```python
from build123d import *

# Parameters (mm, degrees)
SKETCH037_R     = 2.45
PAD019_DEPTH    = 1.6
SKETCH038_R     = 2.45
PAD020_DEPTH    = 1.6
SKETCH062_W     = 1.7771358599
SKETCH062_H     = 3.8
POCKET024_DEPTH = 1.6


with BuildPart() as part:
    # Sketch037 → Pad019 (new body)
    with BuildSketch(Plane.YZ.offset(-8.7)):
        with BuildLine():
            ThreePointArc((-6, 6), (-7.4371881489, -9.1), (-6, -24.2))
            Line((-6, -24.2), (0, -24.2))
            ThreePointArc((0, -24.2), (4.2426406871, -22.4426406871), (6, -18.2))
            Line((6, 0), (6, -18.2))
            ThreePointArc((6, 0), (4.2426406871, 4.2426406871), (0, 6))
            Line((-6, 6), (0, 6))
        make_face()
        Circle(SKETCH037_R, mode=Mode.SUBTRACT)
        with Locations((0, -18.2)):
            Circle(SKETCH037_R, mode=Mode.SUBTRACT)
    extrude(amount=PAD019_DEPTH)

    # Sketch038 → Pad020 (join)
    with BuildSketch(Plane.YZ.offset(-8.7)):
        with BuildLine():
            ThreePointArc((5.8114989668, -16.707860677), (3.6774423219, -13.4590699257), (0, -12.2))
            Line((-7.3771358599, -12.2), (0, -12.2))
            ThreePointArc((-6, 6), (-7.2090239265, -3.0606187573), (-7.3771358599, -12.2))
            Line((-6, 6), (0, 6))
            ThreePointArc((6, 0), (4.2426406871, 4.2426406871), (0, 6))
            Line((6, 0), (6, -17.4420237293))
            Line((6, -17.4420237293), (5.8114989668, -16.707860677))
        make_face()
        Circle(SKETCH038_R, mode=Mode.SUBTRACT)
    extrude(amount=-PAD020_DEPTH)

    # Sketch062 → Pocket024 (cut, symmetric)
    with BuildSketch(Plane.YZ.offset(-8.7)):
        with BuildLine():
            ThreePointArc((-6.3244944235, -22.4), (-6.167388681, -23.3009268767), (-6, -24.2))
            Line((-6, -24.2), (-4.8, -24.2))
            Line((-4.8, -24.2), (-4.8, -22.4))
            Line((-4.8, -22.4), (-6.3244944235, -22.4))
        make_face()
        with Locations((-5.68856793, -9.1)):
            Rectangle(SKETCH062_W, SKETCH062_H)
        with BuildLine():
            Line((-6, 6), (-4.8, 6))
            Line((-4.8, 6), (-4.8, 4.2))
            Line((-4.8, 4.2), (-6.3244944235, 4.2))
            ThreePointArc((-6, 6), (-6.167388681, 5.1009268767), (-6.3244944235, 4.2))
        make_face()
    extrude(amount=POCKET024_DEPTH, both=True, mode=Mode.SUBTRACT)


with BuildPart() as part_1:
    # Body017 placement: moved
    add(part.part.moved(Location((0, -72.6064407756, 0))))


solid = part_1.part
```
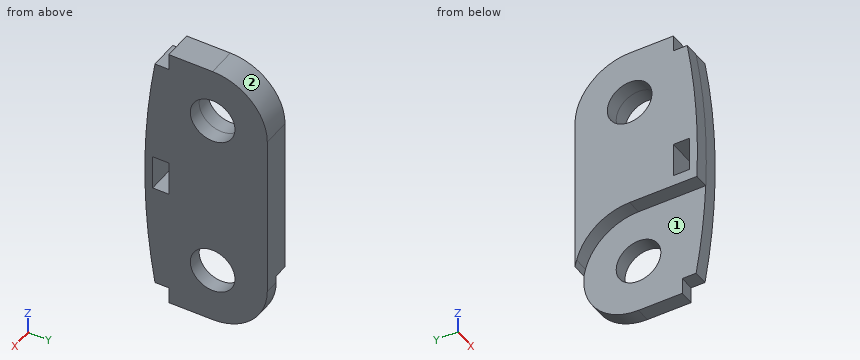
Check sheet for the modelled part. Datum: model origin and axes. Units: mm. Face numbers are marked on the shaded views. A direction names the side the tool comes from. Give positions to 0.01 mm unless a question says otherwise; leave off trailing zeros. Loops run counter-clockwise (first coordinate to the right, second up) from the corner with the lowest first, then second, coordinate; pieces in that order, holes last. Notation, with made-up numbers: (46, 86) - (52, 86) arc R20 cw to (52, 100) - close; hole circle Ø5 at (31.5, 17). An arc over 180 degrees is marked (long way). One line per question, with ' | ' between items. Start each with the question number.
1. Cross-section at A-A, the plane y = -78.5. Enter the section's corners in (x, z).
2. Material ranges on line 1 along Z through (x, y) = (-10, -78.5); line 2 along Z through (x, y) = (-7.6, -78.75); line 3 along Y through (x, z) = (-7.8, 1.5), recorded low to high. Write a range as [from, to].
3. Cross-section at B-B, the plane x = -9.8. Enter the section's corners in (y, z).
4. Set-up check for the marked faces 1 and 2: record each of +Z, -Z, +X, -X, +Y, -Y from which the full face is reachable in a straight line by a thin tool's end or side.
5. Cross-section at C-C, the plane x = -7.85. Enter the section's corners in (y, z), plus the area to 3 significant figures.
6. Gauge pin test, flat ends, axial feed: pin 1 Ø1.8 at (x, z) = (-8, -23) entering from -Y; pin 2 Ø1.4 at (x, y) = (-9, -78.5) entering from -Z; pin 3 Ø0.8 at (x, y) = (-9.5, -75) entering from -Z. Record the tip position at first contact, or that the pin passes through.
7. Cross-section at D-D, the plane y = -71.25. Enter the section's corners in (x, z), plus the area to 3 significant figures.
Check result:
1) outline: (-10.3, -12.2) - (-8.7, -12.2) - (-8.7, -22.4) - (-7.1, -22.4) - (-7.1, -11) - (-10.3, -11) - close; (-10.3, -7.2) - (-7.1, -7.2) - (-7.1, 4.2) - (-10.3, 4.2) - close
2) line 1: z = [-12.2, -11], [-7.2, 4.2] | line 2: z = [-22.4, -11], [-7.2, 4.2] | line 3: y = [-79.34, -74.54], [-70.67, -66.8]
3) outline: (-79.98, -12.2) - (-72.61, -12.2) arc R6 cw to (-66.79, -16.71) - (-66.61, -17.44) - (-66.61, 0) arc R6 ccw to (-72.61, 6) - (-77.41, 6) - (-77.41, 4.2) - (-78.93, 4.2) arc R80.04 ccw to start; hole (-79.18, -11) - (-77.41, -11) - (-77.41, -7.2) - (-79.18, -7.2) - close; hole circle Ø4.9 at (-72.61, 0)
4) face 1: -Z, -X, -Y | face 2: +Z, +X, -X, +Y
5) outline: (-78.93, -22.4) - (-77.41, -22.4) - (-77.41, -24.2) - (-72.61, -24.2) arc R6 ccw to (-66.61, -18.2) - (-66.61, 0) arc R6 ccw to (-72.61, 6) - (-77.41, 6) - (-77.41, 4.2) - (-78.93, 4.2) arc R80.04 ccw to start; hole (-79.18, -11) - (-77.41, -11) - (-77.41, -7.2) - (-79.18, -7.2) - close; hole circle Ø4.9 at (-72.61, -18.2); hole circle Ø4.9 at (-72.61, 0) | area: 327 mm2
6) pin 1: stops at y = -78.98 | pin 2: stops at z = -22.4 | pin 3: stops at z = -12.2
7) outline: (-10.3, -12.36) - (-8.7, -12.36) - (-8.7, -16.16) - (-7.1, -16.16) - (-7.1, -2.04) - (-10.3, -2.04) - close; (-10.3, 2.04) - (-7.1, 2.04) - (-7.1, 5.84) - (-10.3, 5.84) - close; (-8.7, -24.04) - (-7.1, -24.04) - (-7.1, -20.24) - (-8.7, -20.24) - close | area: 57.4 mm2
